from build123d import *

# Parameters (mm, degrees)
CROQUIS1_W              = 36
CROQUIS1_H              = 50
SALIENTE_EXTRUIR1_DEPTH = 3.5
CROQUIS2_R              = 1.1
CORTAR_EXTRUIR2_DEPTH   = 5
CROQUIS5_W              = 3.5
CROQUIS5_H              = 20
CROQUIS5_W_2            = 5.5
CROQUIS5_H_2            = 3.5
SALIENTE_EXTRUIR3_DEPTH = 50
REDONDEO1_R             = 4
CROQUIS6_R              = 2.25
CORTAR_EXTRUIR3_DEPTH   = 2
CROQUIS8_R              = 2.5
CORTAR_EXTRUIR4_DEPTH   = 57.868268832


with BuildPart() as part:
    # Croquis1 → Saliente-Extruir1 (new body)
    with BuildSketch(Plane.XY):
        Rectangle(CROQUIS1_W, CROQUIS1_H)
    extrude(amount=SALIENTE_EXTRUIR1_DEPTH)

    # Croquis2 → Cortar-Extruir2 (cut)
    with BuildSketch(Plane.XY.offset(3.5)):
        with Locations((-13.5, 20)):
            Circle(CROQUIS2_R)
        with Locations((13.5, 20)):
            Circle(CROQUIS2_R)
        with Locations((13.5, 12)):
            Circle(CROQUIS2_R)
        with Locations((13.5, 4)):
            Circle(CROQUIS2_R)
        with Locations((13.5, -4)):
            Circle(CROQUIS2_R)
        with Locations((-13.5, 12)):
            Circle(CROQUIS2_R)
        with Locations((-13.5, 4)):
            Circle(CROQUIS2_R)
        with Locations((-13.5, -4)):
            Circle(CROQUIS2_R)
    extrude(amount=-CORTAR_EXTRUIR2_DEPTH, mode=Mode.SUBTRACT)

    # Croquis5 → Saliente-Extruir3 (add, through all)
    with BuildSketch(Plane(origin=(0, 25, 0), x_dir=(1, 0, 0), z_dir=(0, 1, 0))):
        Polygon((-18, 0), (-20, 0), (-23.5, 0), (-23.5, -3.5), (-18, -3.5), align=None)
        with Locations((-21.75, 10)):
            Rectangle(CROQUIS5_W, CROQUIS5_H)
        with Locations((20.75, -1.75)):
            Rectangle(CROQUIS5_W_2, CROQUIS5_H_2)
        with Locations((21.75, 10)):
            Rectangle(CROQUIS5_W, CROQUIS5_H)
    extrude(amount=-SALIENTE_EXTRUIR3_DEPTH)

    # Redondeo1
    redondeo1_edges = [part.edges().sort_by_distance(p)[0] for p in [
        (-23.5, 0, 3.5),
        (23.5, 0, 3.5),
    ]]
    fillet(redondeo1_edges, radius=REDONDEO1_R)

    # Croquis6 → Cortar-Extruir3 (cut)
    with BuildSketch(Plane(origin=(0, 0, 0), x_dir=(-1, 0, 0), z_dir=(0, 0, -1))):
        with Locations((-13.5, 20)):
            Circle(CROQUIS6_R)
        with Locations((13.5, 20)):
            Circle(CROQUIS6_R)
        with Locations((13.5, 12)):
            Circle(CROQUIS6_R)
        with Locations((13.5, 4)):
            Circle(CROQUIS6_R)
        with Locations((13.5, -4)):
            Circle(CROQUIS6_R)
        with Locations((-13.5, 12)):
            Circle(CROQUIS6_R)
        with Locations((-13.5, 4)):
            Circle(CROQUIS6_R)
        with Locations((-13.5, -4)):
            Circle(CROQUIS6_R)
    extrude(amount=-CORTAR_EXTRUIR3_DEPTH, mode=Mode.SUBTRACT)

    # Croquis8 → Cortar-Extruir4 (cut, through all)
    with BuildSketch(Plane(origin=(23.5, 0, 0), x_dir=(0, 0, -1), z_dir=(1, 0, 0))):
        with Locations((10.25, 12.5)):
            Circle(CROQUIS8_R)
        with Locations((10.25, -12.5)):
            Circle(CROQUIS8_R)
    extrude(amount=-CORTAR_EXTRUIR4_DEPTH, mode=Mode.SUBTRACT)


solid = part.part
Could you check a few things on this model? Use its own coordinates, in mm. A direction names the side the tool comes from. Give positions to 0.01 mm unless a question says otherwise; leave off trailing zeros. Order: outer loops, then holes, each group sorted by start corner. A loop starts at its lowest first (then second) coordinate and runs counter-clockwise, first axis right, second up.
Item 1: I'm going to push flat-ended pins straight in: pin 1 (5 mm diameter, centred on x = 13, y = 5, fed in from -Z); pin 2 (3 mm diameter, centred on x = -13.5, y = -4, fed in from +Z); pin 3 (2 mm diameter, centred on x = -14, y = 3.5, fed in from -Z); pin 4 (8 mm diameter, centred on x = -13.5, z = -15.5, fed in from -Y). Where does each tip first touch, or does it pass through?
Item 2: If we mould it in two halves opening along X, with no side actions, what happens to faces 4 (the face through (15, -4, 2)), 5 (the face through (22, 0, -20)), 6 (the face through (22.297, -0.35, 2.359)), 7 (the face through (13.262, 10.926, 2.76))? For each: pulls with the +X half, pulls with the -X half, needs draft (parallel to the pull), parting line crosses it, or undercut.
Item 3: If we section it at B-B, the plane z = -8.75: Write out the boundary of the cut face in (x, y), plus the area to 3 significant figures.
Item 4: If we section it at C-C, the plane y = -17.5: Write out the boundary of the cut face in (x, z).
Item 5: I need wall thicknesses on line 1 (Y direction, x = -13.5, z = 2.7); line 2 (Y direction, x = 13.5, z = 1.3); line 3 (Y direction, x = 21.8, z = -10.25). Which ranges of each line are inside material? Lowest first, please.
Item 6: If we section it at A-A, the plane y = -4: Write out the boundary of the cut face in (x, z).
Item 7: For faces 1 (the face through (-20, 0, -10)), 2 (the face through (12.29, 13.897, 0.986)), 3 (the face through (-14.311, -3.257, 2.76)), which set-ups out of +Z, -Z, +X, -X, +Y, -Y let a thin tool reach every point of the face, with its end or its side?
Item 8: If we section it at D-D, the plane x = -13.5: Count the separate pieces of the cut face and the enclosed holes in it, plus the area to 3 significant figures.
Values:
1. pin 1: stops at z = 0
1. pin 2: stops at z = 3.5
1. pin 3: stops at z = 2
1. pin 4: passes through
2. face 4: undercut
2. face 5: needs draft
2. face 6: pulls with the +X half
2. face 7: undercut
3. outline: (-23.5, -25) - (-20, -25) - (-20, -14.5) - (-23.5, -14.5) - close; (-23.5, -10.5) - (-20, -10.5) - (-20, 10.5) - (-23.5, 10.5) - close; (-23.5, 14.5) - (-20, 14.5) - (-20, 25) - (-23.5, 25) - close; (20, -25) - (23.5, -25) - (23.5, -14.5) - (20, -14.5) - close; (20, -10.5) - (23.5, -10.5) - (23.5, 10.5) - (20, 10.5) - close; (20, 14.5) - (23.5, 14.5) - (23.5, 25) - (20, 25) - close
3. area: 294 mm2
4. outline: (-23.5, -20) - (-20, -20) - (-20, 0) - (20, 0) - (20, -20) - (23.5, -20) - (23.5, -0.5) arc R4 ccw to (19.5, 3.5) - (-19.5, 3.5) arc R4 ccw to (-23.5, -0.5) - close
5. line 1: y = -25 to -5.1, -2.9 to 2.9, 5.1 to 10.9, 13.1 to 18.9, 21.1 to 25
5. line 2: y = -25 to -6.25, -1.75 to 1.75, 6.25 to 9.75, 14.25 to 17.75, 22.25 to 25
5. line 3: y = -25 to -15, -10 to 10, 15 to 25
6. outline: (-23.5, -20) - (-20, -20) - (-20, 0) - (-15.75, 0) - (-15.75, 2) - (-14.6, 2) - (-14.6, 3.5) - (-19.5, 3.5) arc R4 ccw to (-23.5, -0.5) - close; (-12.4, 2) - (-11.25, 2) - (-11.25, 0) - (11.25, 0) - (11.25, 2) - (12.4, 2) - (12.4, 3.5) - (-12.4, 3.5) - close; (14.6, 2) - (15.75, 2) - (15.75, 0) - (20, 0) - (20, -20) - (23.5, -20) - (23.5, -0.5) arc R4 ccw to (19.5, 3.5) - (14.6, 3.5) - close
7. face 1: -Z, +Y, -Y
7. face 2: -Z
7. face 3: +Z, -Z
8. separate pieces: 5
8. enclosed holes: 0
8. area: 126 mm2
